Design review of the part built by this model. Coordinates are the model's own, in mm. A direction names the side the tool comes from. Coordinates: 2 decimals unless noted, no trailing zeros. Write each loop counter-clockwise with the first axis right and the second up, starting at its lowest first coordinate (ties: lowest second). Pieces come first, ordered by that corner, then holes.
Q1. Take a section at C-C (y = -1.5). State how many separate pieces and enclosed holes the cut face has, and give its area (3 significant figures).
Q2. Mouldability with a two-part tool opening along X and no side actions: class faces 3 (the cylindrical face through (80.74, -3.13, 61.76)), 4 (the cylindrical face through (63.559, -3.131, 107.356)), 5 (the flat face through (-2, 0, 87)), 6 (the cylindrical face through (-63.403, -3.131, 107.406)) as pulls with the +X half, pulls with the -X half, needs draft (parallel to the pull), parting line crosses it, or undercut.
Q3. Insertion check: pin 1 (6 mm diameter, centred on x = -60, z = 41, fed in from +Y); pin 2 (8.5 mm diameter, centred on x = -76.2, z = 60.325, fed in from -Y); pin 3 (3 mm diameter, centred on x = -78.5, y = -2, fed in from -Z). Each pin has a flat end and moves straight along its axis. Give the tip position at first contact, or say it passes through.
Q4. For probe 1 along X at (y, z) = (-2, 97); probe 2 along X at (y, z) = (-1.75, 46); probe 3 along Z at (x, y) = (-53.5, -3.5), list the stretches that pass through material, from the lowest coordinate up.
Q5. Take a section at B-B (z = 73.5). Give the boundary of the cut face in (x, y), and give its area (3 significant figures).
Q6. Machinability: for faces 1 (the cylindrical face through (44.601, -3.219, 34.145)), 2 (the cylindrical face through (-80.96, -3.13, 60.53)), which of the approach directions +Z, -Z, +X, -X, +Y, -Y give a long, thin tool a straight path to every point of the face, cutting with its end or side? Answer none if there is none.
Q7. Take a section at D-D (x = -52). Give the boundary of the cut face in (y, z), and give its area (3 significant figures).
```python
from build123d import *

# Parameters (mm, degrees)
F0_R     = 2.5527
F0_R_2   = 4.7625
F0_R_3   = 11.1125
F0_R_4   = 14.2875
F1_DEPTH = 6.35
F3_DEPTH = 25.4


with BuildPart() as f1:
    # F0 (on Front) → F1 (new body)
    with BuildSketch(Plane.XZ):
        with BuildLine():
            ThreePointArc((-94.654118, 86.472687), (-108.076175, 63.182526), (-99.010505, 37.876462))
            Line((-99.010505, 37.876462), (-43.757367, -18.267594))
            ThreePointArc((-43.757367, -18.267594), (-41.627815, -19.810445), (-39.111045, -20.572845))
            Line((-39.111045, -20.572845), (-3.033135, -25.206036))
            ThreePointArc((-3.033135, -25.206036), (0, -25.4), (3.033135, -25.206036))
            Line((3.033135, -25.206036), (39.111045, -20.572845))
            ThreePointArc((39.111045, -20.572845), (41.627815, -19.810445), (43.757367, -18.267594))
            Line((43.757367, -18.267594), (99.010505, 37.876462))
            ThreePointArc((99.010505, 37.876462), (108.076175, 63.182526), (94.654118, 86.472687))
            Line((94.654118, 86.472687), (68.703576, 104.787667))
            ThreePointArc((68.703576, 104.787667), (63.481204, 107.381191), (57.718982, 108.273567))
            Line((57.718982, 108.273567), (-57.718982, 108.273567))
            ThreePointArc((-57.718982, 108.273567), (-63.481204, 107.381191), (-68.703576, 104.787667))
            Line((-68.703576, 104.787667), (-94.654118, 86.472687))
        make_face()
        with Locations((-38.1, -12.7)):
            Circle(F0_R, mode=Mode.SUBTRACT)
        with Locations((-38.1, 12.7)):
            Circle(F0_R, mode=Mode.SUBTRACT)
        with Locations((38.1, -12.7)):
            Circle(F0_R, mode=Mode.SUBTRACT)
        with Locations((38.1, 12.7)):
            Circle(F0_R, mode=Mode.SUBTRACT)
        with Locations((-99.220218, 49.590496)):
            Circle(F0_R, mode=Mode.SUBTRACT)
        with Locations((-76.2, 60.325)):
            Circle(F0_R_2, mode=Mode.SUBTRACT)
        with Locations((-49.944684, 50.769793)):
            Circle(F0_R_3, mode=Mode.SUBTRACT)
        with Locations((-57.718982, 89.223567)):
            Circle(F0_R_3, mode=Mode.SUBTRACT)
        with Locations((-26.9875, 101.923567)):
            Circle(F0_R, mode=Mode.SUBTRACT)
        with Locations((49.944684, 50.769793)):
            Circle(F0_R_3, mode=Mode.SUBTRACT)
        with Locations((0, 69.5325)):
            Circle(F0_R_4, mode=Mode.SUBTRACT)
        with Locations((99.220218, 49.590496)):
            Circle(F0_R, mode=Mode.SUBTRACT)
        with Locations((76.2, 60.325)):
            Circle(F0_R_2, mode=Mode.SUBTRACT)
        with Locations((26.9875, 101.923567)):
            Circle(F0_R, mode=Mode.SUBTRACT)
        with Locations((57.718982, 89.223567)):
            Circle(F0_R_3, mode=Mode.SUBTRACT)
    extrude(amount=F1_DEPTH)

    # F2 (on face) → F3 (cut)
    with BuildSketch(Plane.XZ.offset(6.35)):
        with BuildLine():
            ThreePointArc((-69.893575, 28.948496), (-85.582074, 29.72708), (-99.010505, 37.876462))
            Line((-99.010505, 37.876462), (-99.010505, -25.4))
            Line((-99.010505, -25.4), (99.010505, -25.4))
            Line((99.010505, -25.4), (99.010505, 37.876462))
            ThreePointArc((99.010505, 37.876462), (85.582074, 29.72708), (69.893575, 28.948496))
            Line((69.893575, 28.948496), (46.503678, 33.649677))
            ThreePointArc((46.503678, 33.649677), (44.574094, 34.153667), (42.714559, 34.874379))
            ThreePointArc((42.714559, 34.874379), (0, 44.1325), (-42.714559, 34.874379))
            ThreePointArc((-42.714559, 34.874379), (-44.574094, 34.153667), (-46.503678, 33.649677))
            Line((-46.503678, 33.649677), (-69.893575, 28.948496))
        make_face()
    extrude(amount=-F3_DEPTH, mode=Mode.SUBTRACT)


solid = f1.part
```
Response:
1. separate pieces: 1
1. enclosed holes: 11
1. area: 11,700 mm2
2. face 3: undercut
2. face 4: pulls with the +X half
2. face 5: needs draft
2. face 6: pulls with the -X half
3. pin 1: stops at y = 0
3. pin 2: passes through
3. pin 3: stops at z = 28.33
4. probe 1: x = -79.74 to -65.66, -49.78 to 49.78, 65.66 to 79.74
4. probe 2: x = -104.82 to -59.98, -39.91 to 39.91, 59.98 to 104.82
4. probe 3: z = 32.24 to 40.24, 61.3 to 78.94, 99.5 to 108.27
5. outline: (-105.37, -6.35) - (-13.73, -6.35) - (-13.73, 0) - (-105.37, 0) - close; (13.73, -6.35) - (105.37, -6.35) - (105.37, 0) - (13.73, 0) - close
5. area: 1,160 mm2
6. face 1: -Z, +Y, -Y
6. face 2: +Y, -Y
7. outline: (-6.35, 32.54) - (0, 32.54) - (0, 39.85) - (-6.35, 39.85) - close; (-6.35, 61.69) - (0, 61.69) - (0, 79.7) - (-6.35, 79.7) - close; (-6.35, 98.75) - (0, 98.75) - (0, 108.27) - (-6.35, 108.27) - close
7. area: 221 mm2
